Model file for the job. Use its own axes, mm. A direction names the side the tool comes from. Coordinates: 2 decimals unless noted, no trailing zeros. Loops run counter-clockwise (first coordinate to the right, second up) from the corner with the lowest first, then second, coordinate; pieces in that order, holes last.
from build123d import *

# Parameters (mm, degrees)
SKETCH1_R               = 1.7
BOSS_EXTRUDE1_DEPTH     = 4
BOSS_EXTRUDE2_DEPTH     = 16
CHAMFER1_SIZE           = 2
FILLET1_R               = 2.08
SKETCH4_W               = 3
SKETCH4_H               = 2.145
CUT_EXTRUDE1_DEPTH      = 7
CUT_EXTRUDE1_DEPTH_BACK = 13
CHAMFER2_SIZE           = 1.705
CHAMFER2_SIZE2          = 1.750863319
CHAMFER2_PART_2_SIZE    = 1.705
CHAMFER2_PART_2_SIZE2   = 1.750863319
CUT_EXTRUDE2_DEPTH      = 3
CUT_EXTRUDE3_DEPTH      = 3


with BuildPart() as part:
    # Sketch1 → Boss-Extrude1 (new body)
    with BuildSketch(Plane(origin=(0, 0, 0), x_dir=(1, 0, 0), z_dir=(0, 1, 0))):
        with BuildLine():
            Line((0, 0), (12.869718626, 0))
            ThreePointArc((12.869718626, 0), (15.756469972, -0.917517095), (17.583763834, -3.333333333))
            ThreePointArc((17.583763834, -3.333333333), (22.031407915, -5.942394239), (25.355, -2))
            Line((25.355, -2), (25.355, 8))
            ThreePointArc((25.355, 8), (22.031407915, 11.942394239), (17.583763834, 9.333333333))
            ThreePointArc((17.583763834, 9.333333333), (15.756469972, 6.917517095), (12.869718626, 6))
            Line((12.869718626, 6), (0, 6))
            Line((0, 6), (0, 0))
        make_face()
        with Locations((21.355, -2)):
            Circle(SKETCH1_R, mode=Mode.SUBTRACT)
        with Locations((21.355, 8)):
            Circle(SKETCH1_R, mode=Mode.SUBTRACT)
    extrude(amount=BOSS_EXTRUDE1_DEPTH)

    # Sketch2 → Boss-Extrude2 (add)
    with BuildSketch(Plane.ZY):
        with BuildLine():
            Line((-6, 0), (0, 0))
            Line((0, 0), (0, 2.084))
            Line((0, 2.084), (3.867185515, 8.555128278))
            ThreePointArc((3.867185515, 8.555128278), (4.610527286, 10.193259862), (4.969057957, 11.956066667))
            ThreePointArc((4.969057957, 11.956066667), (4.839751016, 12.337663541), (4.470991835, 12.5))
            Line((4.470991835, 12.5), (3.466507481, 12.5))
            ThreePointArc((3.466507481, 12.5), (3.131355391, 12.371043228), (2.969083828, 12.050692308))
            ThreePointArc((2.969083828, 12.050692308), (-3, 6.659), (-8.969083828, 12.050692308))
            ThreePointArc((-8.969083828, 12.050692308), (-9.131355391, 12.371043228), (-9.466507481, 12.5))
            Line((-9.466507481, 12.5), (-10.470991835, 12.5))
            ThreePointArc((-10.470991835, 12.5), (-10.839751016, 12.337663541), (-10.969057957, 11.956066667))
            ThreePointArc((-10.969057957, 11.956066667), (-10.610527286, 10.193259862), (-9.867185515, 8.555128278))
            Line((-9.867185515, 8.555128278), (-6, 2.084))
            Line((-6, 2.084), (-6, 0))
        make_face()
    extrude(amount=BOSS_EXTRUDE2_DEPTH)

    # Chamfer1
    chamfer1_edges = [part.edges().sort_by_distance(p)[0] for p in [
        (-16, 0, -3),
    ]]
    chamfer(chamfer1_edges, length=CHAMFER1_SIZE)

    # Fillet1
    fillet1_edges = [part.edges().sort_by_distance(p)[0] for p in [
        (0, 4, -3),
    ]]
    fillet(fillet1_edges, radius=FILLET1_R)

    # Sketch4 → Cut-Extrude1 (cut, two sides)
    with BuildSketch(Plane.XY) as cut_extrude1_sk:
        with Locations((-12.5, 4.2165)):
            Rectangle(SKETCH4_W, SKETCH4_H)
        with Locations((-4.5, 4.2165)):
            Rectangle(SKETCH4_W, SKETCH4_H)
    extrude(amount=CUT_EXTRUDE1_DEPTH, mode=Mode.SUBTRACT)
    extrude(cut_extrude1_sk.sketch, amount=-CUT_EXTRUDE1_DEPTH_BACK, mode=Mode.SUBTRACT)

    # Chamfer2
    chamfer2_edges = [part.edges().sort_by_distance(p)[0] for p in [
        (-4.5, 5.289, -7.915327442),
        (-4.5, 5.289, 1.915327442),
    ]]
    chamfer2_side = [part.faces().sort_by_distance(p)[0] for p in [
        (-4.5, 5.289, -3),
    ]]
    chamfer(chamfer2_edges, length=CHAMFER2_SIZE, length2=CHAMFER2_SIZE2, reference=chamfer2_side[0])

    # Chamfer2 part 2
    chamfer2_part_2_edges = [part.edges().sort_by_distance(p)[0] for p in [
        (-12.5, 5.289, -7.915327442),
        (-12.5, 5.289, 1.915327442),
    ]]
    chamfer2_part_2_side = [part.faces().sort_by_distance(p)[0] for p in [
        (-12.5, 5.289, -3),
    ]]
    chamfer(chamfer2_part_2_edges, length=CHAMFER2_PART_2_SIZE, length2=CHAMFER2_PART_2_SIZE2, reference=chamfer2_part_2_side[0])

    # Sketch5 → Cut-Extrude2 (cut)
    with BuildSketch(Plane.ZY.offset(14)):
        with BuildLine():
            Line((4.439002016, 9.716), (4.439002016, 12))
            ThreePointArc((4.439002016, 12), (4.292555407, 12.353553391), (3.939002016, 12.5))
            Line((3.939002016, 12.5), (4.470991835, 12.5))
            ThreePointArc((4.470991835, 12.5), (4.839751016, 12.337663541), (4.969057957, 11.956066667))
            ThreePointArc((4.969057957, 11.956066667), (4.785021047, 10.816868818), (4.439002016, 9.716))
        make_face()
        with BuildLine():
            Line((-9.939002016, 12.5), (-10.470991835, 12.5))
            ThreePointArc((-10.470991835, 12.5), (-10.839751016, 12.337663541), (-10.969057957, 11.956066667))
            ThreePointArc((-10.969057957, 11.956066667), (-10.785021047, 10.816868818), (-10.439002016, 9.716))
            Line((-10.439002016, 9.716), (-10.439002016, 12))
            ThreePointArc((-10.439002016, 12), (-10.292555407, 12.353553391), (-9.939002016, 12.5))
        make_face()
    extrude(amount=-CUT_EXTRUDE2_DEPTH, mode=Mode.SUBTRACT)

    # Sketch6 → Cut-Extrude3 (cut)
    with BuildSketch(Plane.ZY.offset(6)):
        with BuildLine():
            Line((4.470991835, 12.5), (3.939002016, 12.5))
            ThreePointArc((3.939002016, 12.5), (4.292555407, 12.353553391), (4.439002016, 12))
            Line((4.439002016, 12), (4.439002016, 9.716))
            ThreePointArc((4.439002016, 9.716), (4.785021047, 10.816868818), (4.969057957, 11.956066667))
            ThreePointArc((4.969057957, 11.956066667), (4.839751016, 12.337663541), (4.470991835, 12.5))
        make_face()
        with BuildLine():
            Line((-9.939002016, 12.5), (-10.470991835, 12.5))
            ThreePointArc((-10.470991835, 12.5), (-10.839751016, 12.337663541), (-10.969057957, 11.956066667))
            ThreePointArc((-10.969057957, 11.956066667), (-10.785021047, 10.816868818), (-10.439002016, 9.716))
            Line((-10.439002016, 9.716), (-10.439002016, 12))
            ThreePointArc((-10.439002016, 12), (-10.292555407, 12.353553391), (-9.939002016, 12.5))
        make_face()
    extrude(amount=-CUT_EXTRUDE3_DEPTH, mode=Mode.SUBTRACT)


solid = part.part
Q1. Slice it at B-B (y = 8). List the corners of the cut face in (x, z), and give its area (3 significant figures).
Answers:
outline: (-16, -9.54) - (0, -9.54) - (0, -6.78) - (-16, -6.78) - close; (-16, 0.78) - (0, 0.78) - (0, 3.54) - (-16, 3.54) - close
area: 88.2 mm2
Q2. Mould opens along X. For faces 1 (the flat face through (16, 4, -3)), 2 (the flat face through (25.355, 2, -3)), 3 (the cylindrical face through (15.79, 1.97, -6.94)) say: +X half, -X half, draft (parallel to the pull), parting line (faces both ways), or undercut.
Answers:
face 1: draft
face 2: +X half
face 3: undercut
Q3. Drill centre lines: line 1 (X direction, y = 5.5, z = -7.75); line 2 (Z direction, x = 5, y = 1.5); line 3 (Y direction, x = 13.5, z = -2.75). Where is each one in solid material? Low to high.
Answers:
line 1: x = -16 to -14, -11 to -6, -3 to 0
line 2: z = -6 to 0
line 3: y = 0 to 4
Q4. Which spindle directions (+Z, -Z, +X, -X, +Y, -Y) get a long thin tool onto all of the face, cutting with end or side? Do faces 4 (the flat face through (-7.89, 5.36, -7.96)), 5 (the cylindrical face through (-7.888, 10.169, 4.603)), 6 (the flat face through (-5, 5.289, -3)), 7 (the flat face through (-13, 11, -10.439)), 8 (the flat face through (-5, 11, 4.439)). Say none if no direction does.
Answers:
face 4: -Z, -X, -Y
face 5: +Z, +X, -X, -Y
face 6: +Z, -Z
face 7: -Z, +Y, -Y
face 8: +Z, +Y, -Y
Q5. Flat gauge pins, fed straight in: P1, Ø0.5, axis at y = 10.5, z = -10.5, coming from the +X side; P2, Ø5, axis at x = 5.5, y = 4.5, coming from the +Z side; P3, Ø1.5, axis at x = -5, z = -4.5, coming from the +Y side; P4, Ø2.5, axis at x = 21.355, z = 2, coming from the -Y side. Where does each tip first touch, or does it go through?
Answers:
P1: stops at x = 0
P2: stops at z = 0
P3: stops at y = 7.1
P4: passes through
Q6. Slice it at C-C (z = -4). List the corners of the cut face in (x, y) (3 decimals).
Answers:
outline: (-16, 2) - (-14, 0) - (25.355, 0) - (25.355, 4) - (2.08, 4) arc R2.08 cw to (0, 6.08) - (0, 6.743) - (-16, 6.743) - close; hole (-14, 3.144) - (-11, 3.144) - (-11, 5.289) - (-14, 5.289) - close; hole (-6, 3.144) - (-3, 3.144) - (-3, 5.289) - (-6, 5.289) - close
Q7. Slice it at A-A (x = -9). List the corners of the cut face in (y, z).
Answers:
outline: (0, -6) - (2.08, -6) - (8.56, -9.87) arc R8 ccw to (11.96, -10.97) arc R0.5 ccw to (12.5, -10.47) - (12.5, -9.47) arc R0.5 ccw to (12.05, -8.97) arc R6 cw to (12.05, 2.97) arc R0.5 ccw to (12.5, 3.47) - (12.5, 4.47) arc R0.5 ccw to (11.96, 4.97) arc R8 ccw to (8.56, 3.87) - (2.08, 0) - (0, 0) - close
Q8. Slice it at D-D (y = 4.75). List the corners of the cut face in (x, z), and give its area (3 significant figures).
Answers:
outline: (-16, -7.59) - (-14, -7.59) - (-14, 1.59) - (-16, 1.59) - close; (-11, -7.59) - (-6, -7.59) - (-6, 1.59) - (-11, 1.59) - close; (-3, -7.59) - (0, -7.59) - (0, -6) - (0.48, -6) - (0.48, 0) - (0, 0) - (0, 1.59) - (-3, 1.59) - close
area: 94.7 mm2
